The listing builds one solid part. Answer for the finished solid, in the listing's coordinates (mm). Round coordinates to 2 decimals unless told otherwise and drop trailing zeros. Write each loop counter-clockwise with the first axis right and the second up, starting at its lowest first coordinate (ties: lowest second). Pieces come first, ordered by that corner, then holes. Notation, with made-up numbers: (10, 67.25) - (27, 67.25) arc R21 ccw to (27, 87.25) - close; hole circle Ø11 at (-19.5, 62). An arc over 180 degrees is marked (long way). Answer as CSV lines item,"result". Start each with the question number.
Item 1: For a pull along X with two mould halves and no side action, classify faces 1 (the cylindrical face through (-88.165, -32.429, 2.465)), 2 (the flat face through (-3, 3, 0)), 3 (the cylindrical face through (-88.165, 83.571, 2.465)) as pulls with the +X half, pulls with the -X half, needs draft (parallel to the pull), parting line crosses it, or undercut.
Item 2: Straight lines are drawn through the part: line 1 along Y through (x, z) = (-80, 2.6); line 2 along Y through (x, z) = (15, 2.95); line 3 along Y through (x, z) = (-73.5, 1.2). For each, find the intervals that lie inside material, in ascending order. Write a range as [from, to].
Item 3: A cutting plane is placed at A-A on y = -35. Determine the outline of the cut face in (x, z).
Item 4: A flat-ended cylindrical pin translates along its axis: pin 1 (10.5 mm diameter, centred on x = -80, y = 81, fed in from +Z). Find the tip coordinate at first contact, or state that the pin passes through.
Item 5: A cutting plane is placed at C-C on z = 1.25. Determine the outline of the cut face in (x, y), and give its area (3 significant figures).
Item 6: A cutting plane is placed at B-B on x = 15. Determine the outline of the cut face in (y, z).
Item 7: A cutting plane is placed at D-D on y = 81. Determine the outline of the cut face in (x, z), and give its area (3 significant figures).
```python
from build123d import *

# Parameters (mm, degrees)
ESQUISSE1_W             = 400
ESQUISSE1_H             = 360
BOSS_EXTRU_1_DEPTH      = 5
ESQUISSE5_R             = 8.56
ENL_V_MAT_EXTRU_3_DEPTH = 10
ESQUISSE6_R             = 40
ENL_V_MAT_EXTRU_4_DEPTH = 10


with BuildPart() as part:
    # Esquisse1 → Boss.-Extru.1 (new body)
    with BuildSketch(Plane.XY):
        Rectangle(ESQUISSE1_W, ESQUISSE1_H)
    extrude(amount=BOSS_EXTRU_1_DEPTH)

    # Esquisse5 → Enlèv. mat.-Extru.3 (cut)
    with BuildSketch(Plane(origin=(0, 0, 0), x_dir=(-1, 0, 0), z_dir=(0, 0, -1))):
        with Locations((80, 81)):
            Circle(ESQUISSE5_R)
        with Locations((80, -35)):
            Circle(ESQUISSE5_R)
    extrude(amount=-ENL_V_MAT_EXTRU_3_DEPTH, mode=Mode.SUBTRACT)

    # Esquisse6 → Enlèv. mat.-Extru.4 (cut)
    with BuildSketch(Plane(origin=(0, 0, 0), x_dir=(-1, 0, 0), z_dir=(0, 0, -1))):
        with Locations((-15, 47.5)):
            Circle(ESQUISSE6_R)
    extrude(amount=-ENL_V_MAT_EXTRU_4_DEPTH, mode=Mode.SUBTRACT)


solid = part.part
```
Geometry says:
1,face 1,"undercut"
1,face 2,"needs draft"
1,face 3,"undercut"
2,line 1,"y = [-180, -43.56], [-26.44, 72.44], [89.56, 180]"
2,line 2,"y = [-180, 7.5], [87.5, 180]"
2,line 3,"y = [-180, -40.57], [-29.43, 75.43], [86.57, 180]"
3,outline,"(-200, 0) - (-88.56, 0) - (-88.56, 5) - (-200, 5) - close; (-71.44, 0) - (200, 0) - (200, 5) - (-71.44, 5) - close"
4,pin 1,"passes through"
5,outline,"(-200, -180) - (200, -180) - (200, 180) - (-200, 180) - close; hole circle Ø17.12 at (-80, -35); hole circle Ø17.12 at (-80, 81); hole circle Ø80 at (15, 47.5)"
5,area,"139,000 mm^2"
6,outline,"(-180, 0) - (7.5, 0) - (7.5, 5) - (-180, 5) - close; (87.5, 0) - (180, 0) - (180, 5) - (87.5, 5) - close"
7,outline,"(-200, 0) - (-88.56, 0) - (-88.56, 5) - (-200, 5) - close; (-71.44, 0) - (-6.86, 0) - (-6.86, 5) - (-71.44, 5) - close; (36.86, 0) - (200, 0) - (200, 5) - (36.86, 5) - close"
7,area,"1,700 mm^2"
